Design review of the part built by this model. Coordinates are the model's own, in mm. Face numbers are marked on the shaded views. A direction names the side the tool comes from. Give positions to 0.01 mm unless a question says otherwise; leave off trailing zeros. Loops run counter-clockwise (first coordinate to the right, second up) from the corner with the lowest first, then second, coordinate; pieces in that order, holes last.
from build123d import *

# Parameters (mm, degrees)
F1_DEPTH = 10
F3_D     = 5
F3_DEPTH = 8
F3_TIP   = 1.5021515476
F4_R     = 3
F5_DEPTH = 12


with BuildPart() as f1:
    # F0 (on Top) → F1 (new body)
    with BuildSketch(Plane.XY):
        Polygon((2.8867513459, 5), (-2.8867513459, 5), (-5.7735026919, 0), (-2.8867513459, -5), (2.8867513459, -5), (5.7735026919, 0), align=None)
    extrude(amount=F1_DEPTH)

    # F3
    with Locations(Plane.XY.offset(10)):
        with Locations((0, 0)):
            Hole(F3_D / 2, depth=F3_DEPTH)
            with Locations((0, 0, -(F3_DEPTH + F3_TIP / 2))):  # 118° drill point
                Cone(0, F3_D / 2, F3_TIP, mode=Mode.SUBTRACT)

    # F4 (on face) → F5 (join)
    with BuildSketch(Plane(origin=(0, 0, 0), x_dir=(1, 0, 0), z_dir=(0, 0, -1))):
        Circle(F4_R)
    extrude(amount=F5_DEPTH)


solid = f1.part
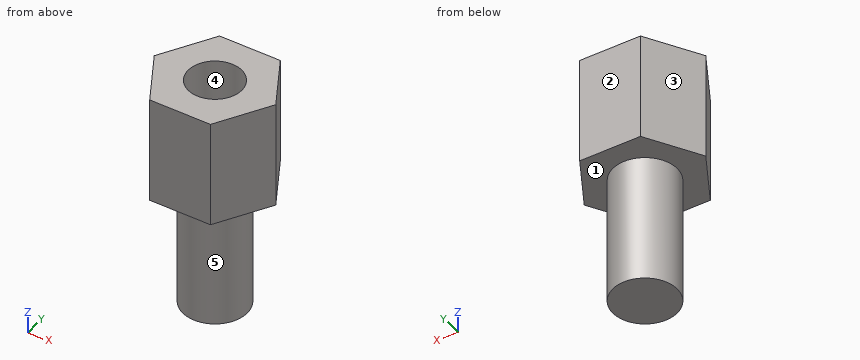
Q1. Draft analysis for pull direction X (two halves, no side actions). For the marked faces 3, 4 and 5, state which applies: pulls with the +X half, pulls with the -X half, needs draft (parallel to the pull), parting line crosses it, or undercut.
Results:
face 3: pulls with the -X half
face 4: undercut
face 5: parting line crosses it
Q2. Tool access review of the marked faces 1 and 2: name each direction out of +Z, -Z, +X, -X, +Y, -Y from which nothing blocks a thin tool from reaching the whole face with its end or side.
Results:
face 1: -Z
face 2: +Z, -Z, +X, -X, +Y
Q3. Take a section at D-D (z = 1.75). Give the boundary of the cut face in (x, y), plus the area to 3 significant figures.
Results:
outline: (-5.77, 0) - (-2.89, -5) - (2.89, -5) - (5.77, 0) - (2.89, 5) - (-2.89, 5) - close; hole circle Ø4.17 at (0, 0)
area: 73.0 mm2
Q4. Take a section at B-B (z = -1). Give the boundary of the cut face in (x, y), plus the area to 3 significant figures.
Results:
outline: circle Ø6 at (0, 0)
area: 28.3 mm2
Q5. Wall thickness on line 1 (Y direction, x = 0, z = 8); line 2 (Z direction, x = 1.5, y = 3.75); line 3 (Y direction, x = -1, z = 7): over which ranges is each line inside the solid? List them lowest first.
Results:
line 1: y = -5 to -2.5, 2.5 to 5
line 2: z = 0 to 10
line 3: y = -5 to -2.29, 2.29 to 5
Q6. Take a section at A-A (z = 4.5). Give the boundary of the cut face in (x, y).
Results:
outline: (-5.77, 0) - (-2.89, -5) - (2.89, -5) - (5.77, 0) - (2.89, 5) - (-2.89, 5) - close; hole circle Ø5 at (0, 0)
Q7. Insertion check: pin 1 (3 mm diameter, centred on y = -1.5, z = -3, fed in from +X); pin 2 (1.5 mm diameter, centred on y = 3.5, z = -2.5, fed in from -X). Each pin has a flat end and moves straight along its axis. Give the tip position at first contact, or say it passes through.
Results:
pin 1: stops at x = 3
pin 2: stops at x = -1.2
Q8. Take a section at C-C (y = 2.75). Give the boundary of the cut face in (x, z), plus the area to 3 significant figures.
Results:
outline: (-4.19, 0) - (-1.2, 0) - (-1.2, -12) - (1.2, -12) - (1.2, 0) - (4.19, 0) - (4.19, 10) - (-4.19, 10) - close
area: 112 mm2
